For this review, take the finished solid that the model builds, in its own axes (mm). A direction names the side the tool comes from. Round coordinates to 2 decimals unless told otherwise and drop trailing zeros. Order: outer loops, then holes, each group sorted by start corner. A loop starts at its lowest first (then second) coordinate and runs counter-clockwise, first axis right, second up. Notation, with made-up numbers: (38, 26) -> (68, 26) arc R29 ccw to (68, 53) -> close; hole circle Ø4 at (61.5, 1). An arc over 180 degrees is marked (long way). Use a Markdown table: item, result. Add a question column.
1) Consider section B-B (z = -79). State the section outline as (x, y) points (3 decimals).
2) Draft analysis for pull direction Y (two halves, no side actions). For faces 4 (the face through (-6.35, -72, -75)), 5 (the face through (-15.875, -141, -41)), 6 (the face through (0, -25.4, -77)), state which applies: pulls with the +Y half, pulls with the -Y half, needs draft (parallel to the pull), parting line crosses it, or undercut.
3) Machinability: for faces 1 (the face through (6.35, -72, -75)), 2 (the face through (15.875, -141, -41)), 3 (the face through (0, -1, -25.4)), which of the approach directions +Z, -Z, +X, -X, +Y, -Y give a long, thin tool a straight path to every point of the face, cutting with its end or side? Answer none if there is none.
4) Wall thickness on line 1 along X through (y, z) = (-67.5, -144) (3 decimals); line 2 along Y through (x, z) = (0, -134); line 3 along X through (y, z) = (12, -19): over which ranges is each line inside the solid? List them lowest first. Write a range as [from, to].
5) Clearance check with flat-ended pins moving along their axes: P1, Ø4, axis at y = -164, z = -56, coming from the -X side (3 decimals); P2, Ø3, axis at y = -76, z = -112, coming from the +X side (3 decimals); P3, Ø3, axis at x = -14, z = -23, coming from the +Y side. State where each tip first meets the part, or that it passes through.
6) Consider section D-D (y = -19). State the section outline as (x, z) points (3 decimals), plus the area to 3 significant figures.
7) Consider section A-A (y = -70.5). State the section outline as (x, z) points (3 decimals).
8) Consider section C-C (z = -134.5). State the section outline as (x, y) points (3 decimals).
```python
from build123d import *
from build123d import SkipClean  # not in build123d's __all__

# Parameters (mm, degrees)
F1_DEPTH = 152.4
F2_DEPTH = 25.4
F4_DEPTH = 31.75
F5_DEPTH = 41.276
F3_W     = 18.2721313551
F3_H     = 101.6
F6_DEPTH = 41.276
F8_DEPTH = 25.4


with BuildPart() as f1:
    # F0 (on Top) → F1 (new body)
    with BuildSketch(Plane.XY):
        with BuildLine():
            ThreePointArc((15.875, -7.1278686449), (8.4122570223, -11.266516889), (0, -12.7))
            ThreePointArc((0, -12.7), (-8.4122570223, -11.266516889), (-15.875, -7.1278686449))
            Line((-15.875, -7.1278686449), (-15.875, -146.8278686449))
            Line((-15.875, -146.8278686449), (15.875, -146.8278686449))
            Line((15.875, -146.8278686449), (15.875, -7.1278686449))
        make_face()
        with BuildLine():
            ThreePointArc((-6.35, -63.5), (-4.4901280605, -59.0098719395), (0, -57.15))
            ThreePointArc((0, -57.15), (4.4901280605, -59.0098719395), (6.35, -63.5))
            Line((6.35, -63.5), (6.35, -114.3))
            ThreePointArc((6.35, -114.3), (0, -120.65), (-6.35, -114.3))
            Line((-6.35, -114.3), (-6.35, -63.5))
        make_face(mode=Mode.SUBTRACT)
        with BuildLine():
            Line((15.875, -7.1278686449), (0, -7.1278686449))
            Line((0, -7.1278686449), (0, -12.7))
            ThreePointArc((0, -12.7), (8.4122570223, -11.266516889), (15.875, -7.1278686449))
        make_face()
        with BuildLine():
            Line((0, -12.7), (0, -7.1278686449))
            Line((0, -7.1278686449), (-15.875, -7.1278686449))
            ThreePointArc((-15.875, -7.1278686449), (-8.4122570223, -11.266516889), (0, -12.7))
        make_face()
    extrude(amount=-F1_DEPTH)

    # F0 (on Top) → F2 (join)
    with BuildSketch(Plane.XY):
        with BuildLine():
            Line((-15.875, -7.1278686449), (0, -7.1278686449))
            Line((0, -7.1278686449), (15.875, -7.1278686449))
            ThreePointArc((15.875, -7.1278686449), (22.8952505992, 1.7014773719), (25.4, 12.7))
            ThreePointArc((25.4, 12.7), (-10.9985226281, 35.5952505992), (-15.875, -7.1278686449))
        make_face()
        with BuildLine():
            ThreePointArc((12.7, 12.7), (8.9802561211, 3.7197438789), (0, 0))
            ThreePointArc((0, 0), (-8.9802561211, 21.6802561211), (12.7, 12.7))
        make_face(mode=Mode.SUBTRACT)
    extrude(amount=-F2_DEPTH)

    # F3 (on face) → F4 (join)
    with BuildSketch(Plane.YZ.offset(15.875)):
        with BuildLine():
            Line((-146.8278686449, -56.3619617548), (-146.8278686449, 0))
            ThreePointArc((-146.8278686449, 0), (-223.0278686449, -76.2), (-146.8278686449, -152.4))
            Line((-146.8278686449, -152.4), (-146.8278686449, -96.0380382452))
            ThreePointArc((-146.8278686449, -96.0380382452), (-152.4, -76.2), (-146.8278686449, -56.3619617548))
        make_face()
    extrude(amount=-F4_DEPTH)

    # F3 (on face) → F5 (cut, through all)
    with BuildSketch(Plane.YZ.offset(15.875)):
        with BuildLine():
            ThreePointArc((-76.2, -76.2), (-103.9971313551, -39.5194752261), (-146.8278686449, -56.3619617548))
            Line((-146.8278686449, -56.3619617548), (-146.8278686449, -96.0380382452))
            ThreePointArc((-146.8278686449, -96.0380382452), (-103.9971313551, -112.8805247739), (-76.2, -76.2))
        make_face()
    with SkipClean():  # cleaning this boolean's faces spoils the solid; the shape is the same uncleaned
        extrude(amount=-F5_DEPTH, mode=Mode.SUBTRACT)

    # F3 (on face) → F6 (cut, through all)
    with BuildSketch(Plane.YZ.offset(15.875)):
        with Locations((-16.2639343225, -76.2)):
            Rectangle(F3_W, F3_H)
    extrude(amount=-F6_DEPTH, mode=Mode.SUBTRACT)

    # F7 (on face) → F8 (join)
    with BuildSketch(Plane(origin=(0, 0, -152.4), x_dir=(1, 0, 0), z_dir=(0, 0, -1))):
        with BuildLine():
            ThreePointArc((-15.875, 7.1278686449), (-10.9985226281, -35.5952505992), (25.4, -12.7))
            ThreePointArc((25.4, -12.7), (22.8952505992, -1.7014773719), (15.875, 7.1278686449))
            Line((15.875, 7.1278686449), (-15.875, 7.1278686449))
        make_face()
        with BuildLine():
            ThreePointArc((0, 0), (8.9802561211, -3.7197438789), (12.7, -12.7))
            ThreePointArc((12.7, -12.7), (-8.9802561211, -21.6802561211), (0, 0))
        make_face(mode=Mode.SUBTRACT)
    extrude(amount=-F8_DEPTH)


solid = f1.part
```
Results list:
| question | item | result |
|---|---|---|
| 1 | outline | (-15.875, -222.976) -> (15.875, -222.976) -> (15.875, -152.297) -> (-15.875, -152.297) -> close; (-15.875, -76.303) -> (-6.35, -76.303) -> (-6.35, -63.5) arc R6.35 cw to (6.35, -63.5) -> (6.35, -76.303) -> (15.875, -76.303) -> (15.875, -25.4) -> (-15.875, -25.4) -> close |
| 2 | face 4 | undercut |
| 2 | face 5 | needs draft |
| 2 | face 6 | pulls with the +Y half |
| 3 | face 1 | +Z, -Z |
| 3 | face 2 | +Z, -Z, +X, -Y |
| 3 | face 3 | +X, -X, +Y |
| 4 | line 1 | [-15.875, -6.35], [6.35, 15.875] |
| 4 | line 2 | [-196.48, -120.65], [-57.15, 0], [25.4, 38.1] |
| 4 | line 3 | [-25.39, -12.68], [12.68, 25.39] |
| 5 | P1 | x = -15.875 |
| 5 | P2 | x = 15.875 |
| 5 | P3 | y = 34.81 |
| 6 | outline | (-15.875, -152.4) -> (15.875, -152.4) -> (15.875, -127) -> (-15.875, -127) -> close; (-15.875, -25.4) -> (15.875, -25.4) -> (15.875, 0) -> (-15.875, 0) -> close |
| 6 | area | 1,610 mm2 |
| 7 | outline | (-15.875, -152.4) -> (-6.35, -152.4) -> (-6.35, 0) -> (-15.875, 0) -> close; (6.35, -152.4) -> (15.875, -152.4) -> (15.875, 0) -> (6.35, 0) -> close |
| 8 | outline | (-15.875, -195.895) -> (15.875, -195.895) -> (15.875, -7.128) arc R25.4 ccw (long way) to (-15.875, -7.128) -> close; hole circle Ø25.4 at (0, 12.7); hole (-6.35, -114.3) arc R6.35 ccw to (6.35, -114.3) -> (6.35, -63.5) arc R6.35 ccw to (-6.35, -63.5) -> close |
